The model under review builds one solid part; all positions refer to its coordinate system, in mm. Face numbers are marked on the shaded views. A direction names the side the tool comes from. Round coordinates to 2 decimals unless told otherwise and drop trailing zeros. Loops run counter-clockwise (first coordinate to the right, second up) from the corner with the lowest first, then second, coordinate; pieces in that order, holes last. Notation, with made-up numbers: M -4,77 L 50,77 A20 ccw 50,88 Z; hole C -21,54.25 d10. An arc over 180 degrees is marked long. Answer as a JSON object with one key per item and string values. Group by question number.
Item 1: Insertion check: P1, Ø1, axis at x = -18, y = 71, coming from the +Z side; P2, Ø0.7, axis at x = -9.5, y = 12, coming from the -Z side; P3, Ø5, axis at x = -1, z = 136, coming from the +Y side. Each pin has a flat end and moves straight along its axis. Give the tip position at first contact, or say it passes through.
Item 2: Tool access review of the marked faces 3 and 4: name each direction out of +Z, -Z, +X, -X, +Y, -Y from which nothing blocks a thin tool from reaching the whole face with its end or side.
Item 3: Consider section D-D (z = 190). Give the boundary of the cut face in (x, y), and give its area (3 significant figures).
Item 4: Consider section A-A (z = 0). Give the boundary of the cut face in (x, y).
Item 5: Consider section C-C (y = 80). Give the boundary of the cut face in (x, z).
Item 6: To check wall thickness, follow line 1 (X direction, y = 12.5, z = 0); line 2 (Y direction, x = -3.5, z = 171.5); line 3 (Y direction, x = 5, z = 62.5). State the ranges of each line that lie inside material, in increasing order.
Item 7: The part is to be moulded in two halves that separate along Z. For the marked faces 1 and 2, say which applies: +Z half, -Z half, draft (parallel to the pull), parting line (faces both ways), or undercut.
Item 8: Consider section B-B (x = 0). Give the boundary of the cut face in (y, z).
```python
from build123d import *

# Parameters (mm, degrees)
CROQUIS4_R                        = 15
CROQUIS4_R_2                      = 7
SALIENTE_EXTRUIR1_DEPTH           = 30
REDONDEO1_R                       = 2
CROQUIS8_W                        = 16.152237462
CROQUIS8_H                        = 16.481036189
SALIENTE_EXTRUIR2_DEPTH           = 26
SALIENTE_EXTRUIR2_TAPER           = -3
SALIENTE_EXTRUIR2_OTHER_WAY_DEPTH = 5
SALIENTE_EXTRUIR2_OTHER_WAY_TAPER = 3
SALIENTE_EXTRUIR4_DEPTH           = 21.4
CORTAR_EXTRUIR2_DEPTH             = 100.8


with BuildPart() as part:
    # Croquis4 → Saliente-Extruir1 (new body)
    with BuildSketch(Plane(origin=(0, 0, 0), x_dir=(1, 0, 0), z_dir=(0, 1, 0))):
        with Locations(Location((0, 0, 0), (0, 0, 270))):
            Circle(CROQUIS4_R)
        with Locations(Location((0, 0, 0), (0, 0, 270))):
            Circle(CROQUIS4_R_2, mode=Mode.SUBTRACT)
    extrude(amount=SALIENTE_EXTRUIR1_DEPTH)

    # Redondeo1
    redondeo1_edges = [part.edges().sort_by_distance(p)[0] for p in [
        (0, 0, -15),
        (0, 30, -15),
    ]]
    fillet(redondeo1_edges, radius=REDONDEO1_R)

    # Croquis8 → Saliente-Extruir2 (add)
    with BuildSketch(Plane.XY.offset(15)):
        with Locations((0.446006576, 14.964559515)):
            Rectangle(CROQUIS8_W, CROQUIS8_H)
    extrude(amount=SALIENTE_EXTRUIR2_DEPTH, taper=SALIENTE_EXTRUIR2_TAPER)

    # Croquis8 → Saliente-Extruir2 other way (add)
    with BuildSketch(Plane.XY.offset(15)):
        with Locations((0.446006576, 14.964559515)):
            Rectangle(CROQUIS8_W, CROQUIS8_H)
    extrude(amount=-SALIENTE_EXTRUIR2_OTHER_WAY_DEPTH, taper=SALIENTE_EXTRUIR2_OTHER_WAY_TAPER)

    # Croquis9 → Saliente-Extruir4 (add, symmetric)
    with BuildSketch(Plane(origin=(0, 0, 0), x_dir=(0, 0, -1), z_dir=(1, 0, 0))):
        Polygon((-41, 24.567679871), (-41, 5.361439159), (-166, 58.420791186), (-166, 77.627031898), align=None)
    extrude(amount=SALIENTE_EXTRUIR4_DEPTH, both=True)

    # Croquis12 → Cortar-Extruir2 (cut, symmetric)
    with BuildSketch(Plane(origin=(0, 50, 0), x_dir=(1, 0, 0), z_dir=(0, 1, 0))):
        Polygon((9.884727568, -41), (13, -166), (33.350069365, -166), (33.350069365, -41), align=None)
    cortar_extruir2 = extrude(amount=CORTAR_EXTRUIR2_DEPTH, both=True, mode=Mode.SUBTRACT)

    # Simetr_a3: Cortar-Extruir2 across plane
    add(cortar_extruir2.mirror(Plane(origin=(0, 0, 0), x_dir=(0, 0, 1), z_dir=(1, 0, 0))), mode=Mode.SUBTRACT)

    # Croquis14 → Revoluci_n1 (revolve)
    with BuildSketch(Plane(origin=(0, 0, 0), x_dir=(0, 0, -1), z_dir=(1, 0, 0)), mode=Mode.PRIVATE) as revoluci_n1_sk:
        Polygon((-190, 85.754128646), (-212, 85.754128646), (-216, 55.754128646), (-190, 55.754128646), align=None)
    revolve(revoluci_n1_sk.sketch.rotate(Axis((0, 79.990867655, 190), (0, 1, 0)), 180), axis=Axis((0, 79.990867655, 190), (0, 1, 0)))


solid = part.part
```
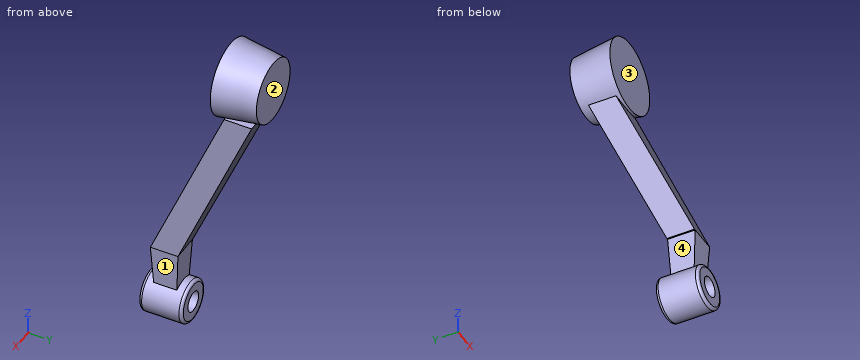
Geometry results:
{
 "1": {"P1": "stops at z = 206.38", "P2": "stops at z = -11.89", "P3": "stops at y = 65.95"},
 "2": {"face 3": "+Z, +X, -X, -Y", "face 4": "-X, +Y, -Y"},
 "3": {"outline": "M -26,55.75 L 26,55.75 L 22,85.75 L -22,85.75 Z", "area": "1,440 mm^2"},
 "4": {"outline": "M -15,2 A2 ccw -13,0 L -7,0 L -7,30 L -13,30 A2 ccw -15,28 Z; M 7,0 L 13,0 A2 ccw 15,2 L 15,28 A2 ccw 13,30 L 7,30 Z"},
 "5": {"outline": "C 0,190 d45.53"},
 "6": {"line 1": "x = -15 to -7, 7 to 15", "line 2": "y = 55.75 to 85.75", "line 3": "y = 14.49 to 33.69"},
 "7": {"face 1": "undercut", "face 2": "draft"},
 "8": {"outline": "M 0,-13 A2 ccw 2,-15 L 28,-15 A2 ccw 30,-13 L 30,-7 L 0,-7 Z; M 0,7 L 30,7 L 30,13 A2 ccw 28,15 L 23.21,15 L 24.57,41 L 77.63,166 L 70.75,166 L 85.75,168 L 85.75,212 L 55.75,216 L 55.75,164 L 57.68,164.26 L 5.36,41 L 6.72,15 L 2,15 A2 ccw 0,13 Z"}
}
